Can you work these out from the model? Positions are in its coordinate system, mm. A direction names the side the tool comes from. Give positions to 0.01 mm unless a question says otherwise; leave off trailing zeros. Order: outer loops, then holes, each group sorted by start corner. A loop starts at its lowest first (then second) coordinate and runs counter-clockwise, first axis right, second up. Notation, with made-up numbers: (21.5, 1.25) - (49.5, 1.25) arc R26 cw to (49.5, 22.25) - close; hole circle Ø5 at (20.5, -3). An arc over 180 degrees is marked (long way). Return JSON: item names as keys, results as strings.
```python
from build123d import *

# Parameters (mm, degrees)
SKETCH1_W           = 11.6713
SKETCH1_H           = 11.43
EXTRUDE1_DEPTH      = 5.83565
EXTRUDE1_DEPTH_BACK = 5.83565
SKETCH2_R           = 5.20065
EXTRUDE2_DEPTH      = 7.9375


with BuildPart() as part:
    # Sketch1 → Extrude1 (new body, two sides)
    with BuildSketch(Plane.XY) as extrude1_sk:
        with Locations((5.83565, 0)):
            Rectangle(SKETCH1_W, SKETCH1_H)
    extrude(amount=EXTRUDE1_DEPTH)
    extrude(extrude1_sk.sketch, amount=-EXTRUDE1_DEPTH_BACK)

    # Sketch2 → Extrude2 (add)
    with BuildSketch(Plane(origin=(11.6713, 0, 0), x_dir=(0, 0, -1), z_dir=(1, 0, 0))):
        Circle(SKETCH2_R)
    extrude(amount=EXTRUDE2_DEPTH)

    # Sketch3 → Revolve1 (revolve)
    with BuildSketch(Plane.XY):
        Polygon((19.6088, 0), (19.6088, 4.064), (20.40255, 4.064), (20.40255, 4.572), (21.99005, 4.572), (21.99005, 0), align=None)
    revolve(axis=Axis((0, 0, 0), (1, 0, 0)))


solid = part.part
```
1. For pin 1 Ø2 at (x, y) = (18.5, -2) entering from -Z; pin 2 Ø4 at (x, z) = (18.5, -2) entering from +Y; pin 3 Ø2 at (x, z) = (15.5, 4) entering from -Y; pin 4 Ø5 at (y, z) = (-4, 3.5) entering from -X, each with a flat end and sliding along its axis, tell me the tip position at first contact or that it passes through.
Checks:
{"pin 1": "z = -5.1", "pin 2": "y = 5.2", "pin 3": "y = -4.25", "pin 4": "x = 0"}
2. Suppose I cut it at A-A (z = 0). List the corners of the cut face in (x, y) for me (3 decimals).
Checks:
{"outline": "(0, -5.715) - (11.671, -5.715) - (11.671, -5.201) - (19.609, -5.201) - (19.609, -4.064) - (20.403, -4.064) - (20.403, -4.572) - (21.99, -4.572) - (21.99, 4.572) - (20.403, 4.572) - (20.403, 4.064) - (19.609, 4.064) - (19.609, 5.201) - (11.671, 5.201) - (11.671, 5.715) - (0, 5.715) - close"}
3. Suppose I cut it at B-B (y = 0). List the corners of the cut face in (x, z) for me, plus the area to 3 significant figures.
Checks:
{"outline": "(0, -5.84) - (11.67, -5.84) - (11.67, -5.2) - (19.61, -5.2) - (19.61, -4.06) - (20.4, -4.06) - (20.4, -4.57) - (21.99, -4.57) - (21.99, 4.57) - (20.4, 4.57) - (20.4, 4.06) - (19.61, 4.06) - (19.61, 5.2) - (11.67, 5.2) - (11.67, 5.84) - (0, 5.84) - close", "area": "240 mm^2"}
4. If I drill on L1, parallel to X at y = -2, z = 4.5; L2, parallel to X at y = -4.25, z = -4.5; L3, parallel to Z at x = 18.75, y = -2.5, over which ranges is the centre line in solid material (lowest first)? Write a range as [from, to].
Checks:
{"L1": "[0, 19.61]", "L2": "[0, 11.67]", "L3": "[-4.56, 4.56]"}
5. On a 3-axis mill with a long thin cutter (end or side, diameter ignored), from which of +Z, -Z, +X, -X, +Y, -Y can I reach the whole of each face in a straight line? I mean faces 1 (the face through (15.584, 4.385, -2.796)), 2 (the face through (19.609, -3, 3)), 3 (the face through (6, -5.715, 0)). Say none if no direction works.
Checks:
{"face 1": "+X", "face 2": "none", "face 3": "+Z, -Z, +X, -X, -Y"}
6. Suppose I cut it at C-C (x = 17.75). List the corners of the cut face in (y, z) for me.
Checks:
{"outline": "circle Ø10.4 at (0, 0)"}
7. Thinking about a two-plate mould opening in X: for faces 4 (the face through (20.011, -0.881, -3.967)), 5 (the face through (11.671, -5.2, 1.4)), 6 (the face through (0, 0, 0)), which applies, +X half, -X half, draft (parallel to the pull), parting line (faces both ways), or undercut?
Checks:
{"face 4": "undercut", "face 5": "+X half", "face 6": "-X half"}
